Source: CAD feature listing. Evaluate the final solid. Frame: model axes, mm. Face numbers are marked on the shaded views. A direction names the side the tool comes from. Round coordinates to 2 decimals unless told otherwise and drop trailing zeros. Loops run counter-clockwise (first coordinate to the right, second up) from the corner with the lowest first, then second, coordinate; pieces in that order, holes last.
(1) Material intervals for probe 1 along Z at (x, y) = (25, 296.5); probe 2 along X at (y, z) = (387.5, 123.5); probe 3 along Y at (x, z) = (14.5, 60), sorted ascending.
(2) Section A-A, the plane y = 405.5. Return the cut outline in (x, z).
(3) Set-up query: the marked faces 1, 2 and 3. Return all of +Z, -Z, +X, -X, +Y, -Y with unobstructed straight access to the full face (end or side cutting, diameter ignored); none if empty.
(4) Mould query, pull axis Z, two halves, no side actions, for the marked faces 4, 5 and 6. Classes: pulls with the +Z half, pulls with the -Z half, needs draft (parallel to the pull), parting line crosses it, or undercut.
(5) First-contact query: pin 1 Ø13 at (y, z) = (192, 136.5) entering from -X; pin 2 Ø4 at (x, y) = (57, 309.5) entering from +Z; pin 3 Ø4 at (y, z) = (406, 70) entering from +X; pin 4 Ø1.5 at (y, z) = (191, 87) entering from -X. Flat tips, straight axial feed; report the tip coordinate or a pass-through.
```python
from build123d import *

# Parameters (mm, degrees)
BOSS_EXTRUDE1_DEPTH = 150
FILLET1_R           = 10
SHELL1_START        = 10
SHELL1_DEPTH        = 130
CUT_EXTRUDE1_REACH  = 525.454
CUT_EXTRUDE2_REACH  = 525.454
SKETCH3_W           = 130
SKETCH3_H           = 190
CUT_EXTRUDE3_REACH  = 523.636
SKETCH5_R           = 3.25
SKETCH6_R           = 2
BOSS_EXTRUDE2_DEPTH = 85
CUT_EXTRUDE4_REACH  = 525.454
BOSS_EXTRUDE3_REACH = 522.676
SKETCH9_W           = 10.749668542
SKETCH9_H           = 9.117335181
SKETCH10_R          = 2
CUT_EXTRUDE6_DEPTH  = 5
SKETCH11_R          = 1.5
CUT_EXTRUDE7_DEPTH  = 5


# Read off the part's stored shape, not the designer's step: Shell1
with BuildPart() as part:
    # Sketch1 → Boss-Extrude1 (new body)
    with BuildSketch(Plane.XY):
        with BuildLine():
            Line((0, 200), (0, 491.430499628))
            Line((0, 491.430499628), (100, 491.430499628))
            ThreePointArc((100, 491.430499628), (64.644660941, 476.785838687), (50, 441.430499628))
            Line((50, 441.430499628), (50, 343.917255306))
            ThreePointArc((50, 343.917255306), (55.711486428, 310.074107136), (72.213286827, 279.979749876))
            ThreePointArc((72.213286827, 279.979749876), (92.855472654, 242.334565721), (100, 200))
            Line((100, 200), (100, 0))
            Line((100, 0), (0, 0))
            Line((0, 0), (0, 200))
        make_face()
    extrude(amount=BOSS_EXTRUDE1_DEPTH)

    # Fillet1
    fillet1_edges = [part.edges().sort_by_distance(p)[0] for p in [
        (64.644660941, 476.785838687, 0),
        (50, 392.673877467, 0),
        (55.711486428, 310.074107136, 0),
        (92.855472654, 242.334565721, 0),
        (100, 100, 0),
        (100, 100, 150),
        (92.855472654, 242.334565721, 150),
        (55.711486428, 310.074107136, 150),
        (50, 392.673877467, 150),
        (64.644660941, 476.785838687, 150),
        (0, 245.715249814, 150),
        (0, 245.715249814, 0),
    ]]
    fillet(fillet1_edges, radius=FILLET1_R)

    # Shell1 outline → Shell1 (cut)
    with BuildSketch(Plane.XY.offset(SHELL1_START)):
        with BuildLine():
            Line((10, 10), (90, 10))
            Line((90, 10), (90, 200))
            ThreePointArc((90, 200), (83.409320496, 239.052766003), (64.367328706, 273.779673977))
            ThreePointArc((64.367328706, 273.779673977), (46.265334269, 306.792307417), (40, 343.917255306))
            Line((40, 343.917255306), (40, 441.430499628))
            ThreePointArc((40, 441.430499628), (47.132359263, 469.803242937), (66.833752096, 491.430499628))
            Line((66.833752096, 491.430499628), (10, 491.430499628))
            Line((10, 491.430499628), (10, 10))
        make_face()
    extrude(amount=SHELL1_DEPTH, mode=Mode.SUBTRACT)

    # Sketch2 → Cut-Extrude1 (cut, up to next)
    with BuildSketch(Plane(origin=(100, 0, 0), x_dir=(0, 0, -1), z_dir=(1, 0, 0)), mode=Mode.PRIVATE) as cut_extrude1_sk1:
        with BuildLine():
            Line((-91.151768807, 184.227304536), (-58.848231193, 184.227304536))
            ThreePointArc((-58.848231193, 184.227304536), (-52.848231193, 178.227304536), (-58.848231193, 172.227304536))
            Line((-58.848231193, 172.227304536), (-91.151768807, 172.227304536))
            ThreePointArc((-91.151768807, 172.227304536), (-97.151768807, 178.227304536), (-91.151768807, 184.227304536))
        make_face()
    cut_extrude1_tool1 = extrude(cut_extrude1_sk1.sketch, amount=-CUT_EXTRUDE1_REACH, mode=Mode.PRIVATE) & part.part
    add(cut_extrude1_tool1.solids().sort_by_distance((100, 178.227305, 75))[0], mode=Mode.SUBTRACT)

    # Sketch3 → Cut-Extrude2 (cut, up to next)
    with BuildSketch(Plane.ZY, mode=Mode.PRIVATE) as cut_extrude2_sk1:
        with Locations((75, 105)):
            Rectangle(SKETCH3_W, SKETCH3_H)
    cut_extrude2_tool1 = extrude(cut_extrude2_sk1.sketch, amount=-CUT_EXTRUDE2_REACH, mode=Mode.PRIVATE) & part.part
    add(cut_extrude2_tool1.solids().sort_by_distance((0, 105, 75))[0], mode=Mode.SUBTRACT)

    # Sketch5 → Cut-Extrude3 (cut, up to next)
    with BuildSketch(Plane.ZY.offset(-90), mode=Mode.PRIVATE) as cut_extrude3_sk1:
        with Locations((40, 18)):
            Circle(SKETCH5_R)
    cut_extrude3_tool1 = extrude(cut_extrude3_sk1.sketch, amount=-CUT_EXTRUDE3_REACH, mode=Mode.PRIVATE) & part.part
    # Sketch5 → Cut-Extrude3 (cut, up to next)
    with BuildSketch(Plane.ZY.offset(-90), mode=Mode.PRIVATE) as cut_extrude3_sk2:
        with Locations((110, 18)):
            Circle(SKETCH5_R)
    cut_extrude3_tool2 = extrude(cut_extrude3_sk2.sketch, amount=-CUT_EXTRUDE3_REACH, mode=Mode.PRIVATE) & part.part
    add(cut_extrude3_tool1.solids().sort_by_distance((90, 18, 40))[0], mode=Mode.SUBTRACT)
    add(cut_extrude3_tool2.solids().sort_by_distance((90, 18, 110))[0], mode=Mode.SUBTRACT)

    # Sketch6 → Boss-Extrude2 (add)
    # profile 1 of 4: a face of its own
    with BuildSketch(Plane.ZY.offset(-90)):
        with BuildLine():
            Line((10, 200), (10, 188))
            ThreePointArc((10, 188), (18.485281374, 191.514718626), (22, 200))
            Line((22, 200), (10, 200))
        make_face()
        with Locations((14.732857766, 195.683462966)):
            Circle(SKETCH6_R, mode=Mode.SUBTRACT)
    # profile 2 of 4: a face of its own
    with BuildSketch(Plane.ZY.offset(-90)):
        with BuildLine():
            Line((140, 200), (140, 188))
            ThreePointArc((140, 188), (131.514718626, 191.514718626), (128, 200))
            Line((128, 200), (140, 200))
        make_face()
        with Locations(Location((135.267142234, 195.683462966, 0), (0, 0, 180))):
            Circle(SKETCH6_R, mode=Mode.SUBTRACT)
    # profile 3 of 4: a face of its own
    with BuildSketch(Plane.ZY.offset(-90)):
        with BuildLine():
            Line((140, 10), (128, 10))
            ThreePointArc((128, 10), (131.514718626, 18.485281374), (140, 22))
            Line((140, 22), (140, 10))
        make_face()
        with Locations((135.267142234, 14.316537034)):
            Circle(SKETCH6_R, mode=Mode.SUBTRACT)
    # profile 4 of 4: a face of its own
    with BuildSketch(Plane.ZY.offset(-90)):
        with BuildLine():
            Line((10, 10), (22, 10))
            ThreePointArc((22, 10), (18.485281374, 18.485281374), (10, 22))
            Line((10, 22), (10, 10))
        make_face()
        with Locations(Location((14.732857766, 14.316537034, 0), (0, 0, 180))):
            Circle(SKETCH6_R, mode=Mode.SUBTRACT)
    extrude(amount=BOSS_EXTRUDE2_DEPTH)

    # Sketch8 → Cut-Extrude4 (cut, up to next)
    with BuildSketch(Plane(origin=(0, 0, 0), x_dir=(-1, 0, 0), z_dir=(0, 0, -1)), mode=Mode.PRIVATE) as cut_extrude4_sk1:
        Polygon((-64.644660941, 476.785838687), (-79.289321881, 491.430499628), (-115.095354781, 491.430499628), align=None)
    cut_extrude4_tool1 = extrude(cut_extrude4_sk1.sketch, amount=-CUT_EXTRUDE4_REACH, mode=Mode.PRIVATE) & part.part
    add(cut_extrude4_tool1.solids().sort_by_distance((86.343113, 486.548946, 0))[0], mode=Mode.SUBTRACT)

    # Sketch9 → Boss-Extrude3 (add, up to next)
    with BuildSketch(Plane.XY.offset(10), mode=Mode.PRIVATE) as boss_extrude3_sk1:
        Polygon((22.020157431, 491.430499628), (10, 480.807276536), (10, 491.430499628), align=None)
    boss_extrude3_tool1 = extrude(boss_extrude3_sk1.sketch, amount=BOSS_EXTRUDE3_REACH, mode=Mode.PRIVATE) - part.part
    # Sketch9 → Boss-Extrude3 (add, up to next)
    with BuildSketch(Plane.XY.offset(10), mode=Mode.PRIVATE) as boss_extrude3_sk2:
        with Locations((61.458917825, 486.871832037)):
            Rectangle(SKETCH9_W, SKETCH9_H)
    boss_extrude3_tool2 = extrude(boss_extrude3_sk2.sketch, amount=BOSS_EXTRUDE3_REACH, mode=Mode.PRIVATE) - part.part
    add(boss_extrude3_tool1.solids().sort_by_distance((14.006719, 487.889425, 10))[0])
    add(boss_extrude3_tool2.solids().sort_by_distance((61.458918, 486.871832, 10))[0])

    # Sketch10 → Cut-Extrude6 (cut)
    with BuildSketch(Plane(origin=(0, 491.430499628, 0), x_dir=(1, 0, 0), z_dir=(0, 1, 0))):
        with Locations(Location((13.117335181, -15, 0), (0, 0, 270))):
            Circle(SKETCH10_R)
        with Locations(Location((62.947163257, -15.024173332, 0), (0, 0, 270))):
            Circle(SKETCH10_R)
        with Locations(Location((62.860866202, -135.163680398, 0), (0, 0, 270))):
            Circle(SKETCH10_R)
        with Locations(Location((13.087879919, -135.163680398, 0), (0, 0, 270))):
            Circle(SKETCH10_R)
    extrude(amount=-CUT_EXTRUDE6_DEPTH, mode=Mode.SUBTRACT)

    # Sketch11 → Cut-Extrude7 (cut)
    with BuildSketch(Plane.ZY.offset(-90)):
        with Locations((87.434890577, 190.781669354)):
            Circle(SKETCH11_R)
        with Locations((63.434890577, 190.449058246)):
            Circle(SKETCH11_R)
        with Locations((63.767501685, 166.449058246)):
            Circle(SKETCH11_R)
        with Locations((87.767501685, 166.781669354)):
            Circle(SKETCH11_R)
    extrude(amount=-CUT_EXTRUDE7_DEPTH, mode=Mode.SUBTRACT)


solid = part.part
```
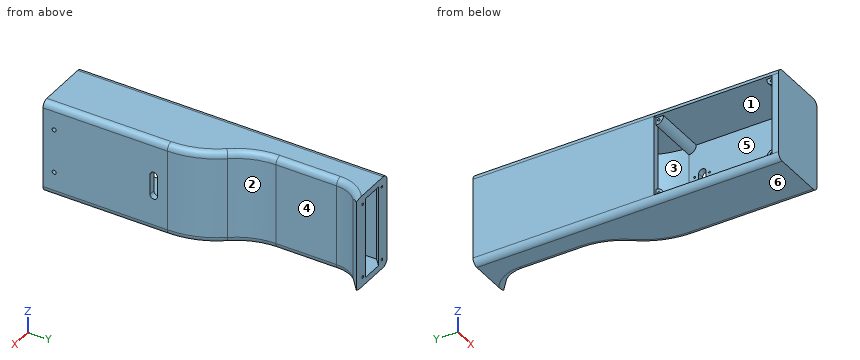
Output values:
1. probe 1: z = 0 to 10, 140 to 150
1. probe 2: x = 0 to 10, 40 to 50
1. probe 3: y = 0 to 10, 484.78 to 491.43
2. outline: (0, 10) arc R10 ccw to (10, 0) - (40, 0) arc R10 ccw to (50, 10) - (50, 140) arc R10 ccw to (40, 150) - (10, 150) arc R10 ccw to (0, 140) - close; hole (10, 10) - (40, 10) - (40, 140) - (10, 140) - close
3. face 1: -X
3. face 2: +Z, -Z, +X
3. face 3: none
4. face 4: needs draft
4. face 5: undercut
4. face 6: pulls with the -Z half
5. pin 1: stops at x = 0
5. pin 2: stops at z = 144.31
5. pin 3: stops at x = 50
5. pin 4: stops at x = 95
